Autodesk Inventor part; units mm, degrees
ref_plane "YZ Plane" through (0, 0, 0) normal (1, 0, 0) x (0, 1, 0)
ref_plane "XZ Plane" through (0, 0, 0) normal (0, 1, 0) x (-1, 0, 0)
ref_plane "XY Plane" through (0, 0, 0) normal (0, 0, 1) x (1, 0, 0)
sketch "Skizze1" plane through (0, 0, 0) normal (0, 0, 1) x (1, 0, 0)
  line L0 (0, 0) -> (0, 20.7958)
  line L1 (0, 20.7958) -> (40, 25)
  line L2 (40, 25) -> (405, 25)
  line L3 (405, 25) -> (405, 0)
  line L4 (405, 0) -> (0, 0)
  line L5 (405, 0) -> (435, 0)
  line L6 (435, 0) -> (435, 20)
  line L7 (435, 20) -> (405, 20)
  line L8 (405, 20) -> (405, 0)
  line L9 (435, 15) -> (480, 15)
  line L10 (480, 15) -> (480, -15)
  line L11 (480, -15) -> (435, -15)
  line L12 (435, -15) -> (435, 15)
  dimension "d0" = 480
  dimension "d1" = 30
  dimension "d2" = 40
  dimension "d3" = 50
  dimension "d4" = 6
  dimension "d5" = 40
  dimension "d6" = 30
  dimension "d7" = 75
revolve "Umdrehung1" add sketch "Skizze1" angle 360 about axis through (405, 0, 0) along (-1, 0, 0) contours L0 L1 L2 L3 L4 | L3 L7 L6 L5
extrude "Extrusion1" add sketch "Skizze1" along normal mid plane 24 contours L6 L9 L10 L11 L12
full round fillet "Rundung1" first side at (450, 15, 4) centre faces at (480, 5, 4) second side at (450, -15, -4)
extrude "Extrusion2" cut sketch "Skizze1" along normal mid plane 8 contours L6 L9 L10 L11 L12
sketch "Skizze2" plane through (0, 0, 12) normal (0, 0, 1) x (1, 0, 0)
  arc A0 (465, -15) -> (465, 15) centre (465, 0) ccw
  point P0 (0, 0)
hole "Bohrung1" at (465, 0, 12) direction (0, 0, -1) diameter 14 end through all
sketch "Skizze3" plane through (435, 0, 0) normal (1, 0, 0) x (0, 0, -1)
  line L0 (-15, -20) -> (-20, -20)
  line L1 (-20, -20) -> (-20, 20)
  line L2 (-20, 20) -> (-15, 20)
  line L3 (-15, 20) -> (-15, -20)
  line L4 (20, -20) -> (15, -20)
  line L5 (15, -20) -> (15, 20)
  line L6 (15, 20) -> (20, 20)
  line L7 (20, 20) -> (20, -20)
  circle A0 centre (0, 0) radius 20
  point P0 (-15, -13.2288)
  point P1 (-20, 0)
  point P2 (-15, 13.2288)
  dimension "d20" = 30
extrude "Extrusion3" cut sketch "Skizze3" against normal up to surface (30 mm away) contours L0 L1 A0 L3 | A0 L3 | L1 L2 L3 A0 | A0 L7 L4 L5 | L5 A0 | L5 L6 L7 A0
chamfer "Fase1" distance 2 angle 45 2 edges at (405, -25, 0) (0, -20.7958, 0)
properties part number "Kolbenstange" material "Stahl AISI 4130"
Input: part model. Units: mm. Frame: model coordinates. A direction names the side the tool comes from. Give positions to 0.01 mm unless a question says otherwise; leave off trailing zeros. Order: outer loops, then holes, each group sorted by start corner. A loop starts at its lowest first (then second) coordinate and runs counter-clockwise, first axis right, second up. Notation, with made-up numbers: (18.25, 57.25) -> (59.25, 57.25) arc R15 cw to (59.25, 72.25) -> close; hole circle Ø5 at (22, -9). An arc over 180 degrees is marked (long way). Use one line per item in the form item = value.
1) Mould query, pull axis Z, two halves, no side actions, for faces 1 (the flat face through (457, 0, 12)), 2 (the flat face through (457, 0, 4)), 3 (the conical face through (404.875, 12.432, -19.499)). Classes: pulls with the +Z half, pulls with the -Z half, needs draft (parallel to the pull), parting line crosses it, or undercut.
Response values:
face_1 = pulls with the +Z half
face_2 = undercut
face_3 = parting line crosses it
2) Line query: probe 1 along Y at (x, z) = (465, 8.75); probe 2 along X at (y, z) = (0, 9); probe 3 along X at (y, z) = (-3, -2). Output: solid intervals per line, ascending.
Response values:
probe_1 = -15 to -7, 7 to 15
probe_2 = 0 to 458, 472 to 480
probe_3 = 0 to 435
3) First-contact query: pin 1 Ø4 at (x, y) = (166, -12.5) entering from +Z; pin 2 Ø1 at (x, z) = (386, 8.5) entering from +Y; pin 3 Ø2.5 at (x, z) = (452.5, -8.5) entering from -Y. Flat tips, straight axial feed; report the tip coordinate or a pass-through.
Response values:
pin_1 = 22.69
pin_2 = 23.69
pin_3 = -15
4) Reachability of faces 4 (the flat face through (420, 0, 15)), 5 (the cylindrical face through (420, 20, 0)), 6 (the flat face through (420, 0, -15)), 7 (the flat face through (450, -15, 8)) from +Z, -Z, +X, -X, +Y, -Y: full face, straight path, thin tool, end or side. Return the list, or none.
Response values:
face_4 = +Z, +X, +Y, -Y
face_5 = +X, +Y
face_6 = -Z, +X, +Y, -Y
face_7 = +Z, -Z, +X, -Y
5) Section A-A, the plane z = 0. Return loops of the section in (x, y).
Response values:
outline = (0, -18.8) -> (1.99, -21) -> (40, -25) -> (403, -25) -> (405, -23) -> (405, -20) -> (435, -20) -> (435, 20) -> (405, 20) -> (405, 23) -> (403, 25) -> (40, 25) -> (1.99, 21) -> (0, 18.8) -> close
6) Section B-B, the plane x = 149. Return loops of the section in (y, z), and give its area (3 significant figures).
Response values:
outline = circle Ø50 at (0, 0)
area = 1,960 mm^2
